CAD build for the part. Positions are in the model's coordinates, mm. A direction names the side the tool comes from. Round coordinates to 2 decimals unless told otherwise and drop trailing zeros. Write each loop counter-clockwise with the first axis right and the second up, starting at its lowest first coordinate (ties: lowest second). Pieces come first, ordered by that corner, then holes. Notation, with made-up numbers: (-7.5, 45) - (45.5, 45) arc R21 ccw to (45.5, 73) - close; hole circle Ø10 at (75, -38). An arc over 180 degrees is marked (long way). Use one line per item in the form item = value. Start each with the question number.
Item 1: Band-saw the part on D-D, the plane x = 18. List the corners of the cut face in (y, z).
Item 2: Tool access for faces 1 (the cylindrical face through (0.73, 3.147, 10.015)), 2 (the flat face through (0, 0, 0)): list every direction of +Z, -Z, +X, -X, +Y, -Y with a clear straight run to the whole face (end or side of a thin tool).
Item 3: Drill centre lines: L1, parallel to Z at x = -5, y = 4.25; L2, parallel to Z at x = -6, y = 5.75; L3, parallel to X at y = 1.25, z = 4.5. Where is each one in solid material? Low to high.
Item 4: Band-saw the part on A-A, the plane y = 2.25. Give the number of separate pieces and of enclosed holes in the cut face, and give its area (3 significant figures).
Item 5: Pin check, flat tips, straight feed: pin 1 (1 mm diameter, centred on y = 0.5, z = 11, fed in from +X); pin 2 (2 mm diameter, centred on x = -5, z = 17, fed in from +Y); pin 3 (1 mm diameter, centred on x = 8, y = 3.5, fed in from -Z); pin 4 (1 mm diameter, centred on x = -19, z = 16, fed in from -Y). Stop position of each tip, or through.
from build123d import *

# Parameters (mm, degrees)
SKETCH1_R           = 50.8
BOSS_EXTRUDE1_DEPTH = 25.4
SKETCH2_R           = 69.85
SKETCH2_R_2         = 50.8
BOSS_EXTRUDE2_DEPTH = 12.7
SKETCH3_R           = 49.53
SKETCH3_R_2         = 47.625
CUT_EXTRUDE1_DEPTH  = 1.1176
CUT_EXTRUDE2_REACH  = 27.4
SKETCH4_R           = 3.175
SKETCH5_R           = 11.43
CUT_EXTRUDE3_DEPTH  = 19.05
SKETCH42_OUTSIDE_W  = 181.538
SKETCH42_OUTSIDE_H  = 181.538
SKETCH42_OUTSIDE_R  = 23.8125
CUT_EXTRUDE9_DEPTH  = 30.48
SKETCH43_R          = 20.6375
CUT_EXTRUDE10_DEPTH = 19.05
SKETCH52_R          = 23.8125
CUT_EXTRUDE11_DEPTH = 19.05
SKETCH55_R          = 1.905
CUT_EXTRUDE12_DEPTH = 7.62
CIRPATTERN1_COUNT   = 8
SKETCH58_R          = 0.9525
CUT_EXTRUDE14_DEPTH = 7.62
CIRPATTERN2_COUNT   = 4
SKETCH59_R          = 0.9525
SKETCH59_R_2        = 1.905
INLET_LID_DEPTH     = 0.03175
SKETCH60_R          = 0.9525
SKETCH60_R_2        = 1.905
OUTLET_LID_DEPTH    = 0.0635


with BuildPart() as part:
    # Sketch1 → Boss-Extrude1 (new body)
    with BuildSketch(Plane(origin=(0, 0, 0), x_dir=(1, 0, 0), z_dir=(0, 1, 0))):
        Circle(SKETCH1_R)
    extrude(amount=BOSS_EXTRUDE1_DEPTH)

    # Sketch2 → Boss-Extrude2 (add)
    with BuildSketch(Plane.XZ):
        Circle(SKETCH2_R)
        Circle(SKETCH2_R_2, mode=Mode.SUBTRACT)
    extrude(amount=-BOSS_EXTRUDE2_DEPTH)

    # Sketch3 → Cut-Extrude1 (cut)
    with BuildSketch(Plane.XZ):
        Circle(SKETCH3_R)
        Circle(SKETCH3_R_2, mode=Mode.SUBTRACT)
    extrude(amount=-CUT_EXTRUDE1_DEPTH, mode=Mode.SUBTRACT)

    # Sketch4 → Cut-Extrude2 (cut, up to next)
    with BuildSketch(Plane.XZ, mode=Mode.PRIVATE) as cut_extrude2_sk1:
        with Locations((0, -59.9186)):
            Circle(SKETCH4_R)
    cut_extrude2_tool1 = extrude(cut_extrude2_sk1.sketch, amount=-CUT_EXTRUDE2_REACH, mode=Mode.PRIVATE) & part.part
    add(cut_extrude2_tool1.solids().sort_by_distance((0, 0, -59.9186))[0], mode=Mode.SUBTRACT)
    # Sketch4 → Cut-Extrude2 (cut, up to next)
    with BuildSketch(Plane.XZ, mode=Mode.PRIVATE) as cut_extrude2_sk2:
        with Locations((-42.368848379, -42.368848379)):
            Circle(SKETCH4_R)
    cut_extrude2_tool2 = extrude(cut_extrude2_sk2.sketch, amount=-CUT_EXTRUDE2_REACH, mode=Mode.PRIVATE) & part.part
    add(cut_extrude2_tool2.solids().sort_by_distance((-42.368848, 0, -42.368848))[0], mode=Mode.SUBTRACT)
    # Sketch4 → Cut-Extrude2 (cut, up to next)
    with BuildSketch(Plane.XZ, mode=Mode.PRIVATE) as cut_extrude2_sk3:
        with Locations((-59.9186, 0)):
            Circle(SKETCH4_R)
    cut_extrude2_tool3 = extrude(cut_extrude2_sk3.sketch, amount=-CUT_EXTRUDE2_REACH, mode=Mode.PRIVATE) & part.part
    add(cut_extrude2_tool3.solids().sort_by_distance((-59.9186, 0, 0))[0], mode=Mode.SUBTRACT)
    # Sketch4 → Cut-Extrude2 (cut, up to next)
    with BuildSketch(Plane.XZ, mode=Mode.PRIVATE) as cut_extrude2_sk4:
        with Locations((-42.368848379, 42.368848379)):
            Circle(SKETCH4_R)
    cut_extrude2_tool4 = extrude(cut_extrude2_sk4.sketch, amount=-CUT_EXTRUDE2_REACH, mode=Mode.PRIVATE) & part.part
    add(cut_extrude2_tool4.solids().sort_by_distance((-42.368848, 0, 42.368848))[0], mode=Mode.SUBTRACT)
    # Sketch4 → Cut-Extrude2 (cut, up to next)
    with BuildSketch(Plane.XZ, mode=Mode.PRIVATE) as cut_extrude2_sk5:
        with Locations((0, 59.9186)):
            Circle(SKETCH4_R)
    cut_extrude2_tool5 = extrude(cut_extrude2_sk5.sketch, amount=-CUT_EXTRUDE2_REACH, mode=Mode.PRIVATE) & part.part
    add(cut_extrude2_tool5.solids().sort_by_distance((0, 0, 59.9186))[0], mode=Mode.SUBTRACT)
    # Sketch4 → Cut-Extrude2 (cut, up to next)
    with BuildSketch(Plane.XZ, mode=Mode.PRIVATE) as cut_extrude2_sk6:
        with Locations((42.368848379, 42.368848379)):
            Circle(SKETCH4_R)
    cut_extrude2_tool6 = extrude(cut_extrude2_sk6.sketch, amount=-CUT_EXTRUDE2_REACH, mode=Mode.PRIVATE) & part.part
    add(cut_extrude2_tool6.solids().sort_by_distance((42.368848, 0, 42.368848))[0], mode=Mode.SUBTRACT)
    # Sketch4 → Cut-Extrude2 (cut, up to next)
    with BuildSketch(Plane.XZ, mode=Mode.PRIVATE) as cut_extrude2_sk7:
        with Locations((59.9186, 0)):
            Circle(SKETCH4_R)
    cut_extrude2_tool7 = extrude(cut_extrude2_sk7.sketch, amount=-CUT_EXTRUDE2_REACH, mode=Mode.PRIVATE) & part.part
    add(cut_extrude2_tool7.solids().sort_by_distance((59.9186, 0, 0))[0], mode=Mode.SUBTRACT)
    # Sketch4 → Cut-Extrude2 (cut, up to next)
    with BuildSketch(Plane.XZ, mode=Mode.PRIVATE) as cut_extrude2_sk8:
        with Locations((42.368848379, -42.368848379)):
            Circle(SKETCH4_R)
    cut_extrude2_tool8 = extrude(cut_extrude2_sk8.sketch, amount=-CUT_EXTRUDE2_REACH, mode=Mode.PRIVATE) & part.part
    add(cut_extrude2_tool8.solids().sort_by_distance((42.368848, 0, -42.368848))[0], mode=Mode.SUBTRACT)

    # Sketch5 → Cut-Extrude3 (cut)
    with BuildSketch(Plane(origin=(0, 25.4, 0), x_dir=(1, 0, 0), z_dir=(0, 1, 0))):
        Circle(SKETCH5_R)
    extrude(amount=-CUT_EXTRUDE3_DEPTH, mode=Mode.SUBTRACT)

    # Sketch42 outside → Cut-Extrude9 (cut)
    with BuildSketch(Plane.XZ):
        Rectangle(SKETCH42_OUTSIDE_W, SKETCH42_OUTSIDE_H)
        Circle(SKETCH42_OUTSIDE_R, mode=Mode.SUBTRACT)
    extrude(amount=-CUT_EXTRUDE9_DEPTH, mode=Mode.SUBTRACT)

    # Sketch43 → Cut-Extrude10 (cut)
    with BuildSketch(Plane(origin=(0, 25.4, 0), x_dir=(1, 0, 0), z_dir=(0, 1, 0))):
        Circle(SKETCH43_R)
    extrude(amount=-CUT_EXTRUDE10_DEPTH, mode=Mode.SUBTRACT)

    # Sketch52 → Cut-Extrude11 (cut)
    with BuildSketch(Plane(origin=(0, 25.4, 0), x_dir=(1, 0, 0), z_dir=(0, 1, 0))):
        Circle(SKETCH52_R)
    extrude(amount=-CUT_EXTRUDE11_DEPTH, mode=Mode.SUBTRACT)

    # Sketch55 → Cut-Extrude12 (cut)
    with BuildSketch(Plane.XZ):
        with Locations((8.255, 0)):
            Circle(SKETCH55_R)
    cut_extrude12 = extrude(amount=-CUT_EXTRUDE12_DEPTH, mode=Mode.SUBTRACT)

    # CirPattern1: Cut-Extrude12 ×8 about axis
    cirpattern1_axis = Axis((0, 0, 0), (0, 1, 0))
    for i in range(1, CIRPATTERN1_COUNT):
        add(cut_extrude12.rotate(cirpattern1_axis, i * 360 / CIRPATTERN1_COUNT), mode=Mode.SUBTRACT)

    # Sketch58 → Cut-Extrude14 (cut)
    with BuildSketch(Plane.XZ):
        with Locations((3.175, 0)):
            Circle(SKETCH58_R)
    cut_extrude14 = extrude(amount=-CUT_EXTRUDE14_DEPTH, mode=Mode.SUBTRACT)

    # CirPattern2: Cut-Extrude14 ×4 about axis
    cirpattern2_axis = Axis((0, 0, 0), (0, 1, 0))
    for i in range(1, CIRPATTERN2_COUNT):
        add(cut_extrude14.rotate(cirpattern2_axis, i * 360 / CIRPATTERN2_COUNT), mode=Mode.SUBTRACT)

    # Sketch59 → Inlet Lid (add, symmetric)
    with BuildSketch(Plane(origin=(0, 6.35, 0), x_dir=(1, 0, 0), z_dir=(0, 1, 0))):
        with Locations((0, -3.175)):
            Circle(SKETCH59_R)
        with Locations((-3.175, 0)):
            Circle(SKETCH59_R)
        with Locations((0, 3.175)):
            Circle(SKETCH59_R)
        with Locations((3.175, 0)):
            Circle(SKETCH59_R)
        with Locations((0, 8.255)):
            Circle(SKETCH59_R_2)
        with Locations((-5.837166479, 5.837166479)):
            Circle(SKETCH59_R_2)
        with Locations((-8.255, 0)):
            Circle(SKETCH59_R_2)
        with Locations((-5.837166479, -5.837166479)):
            Circle(SKETCH59_R_2)
        with Locations((0, -8.255)):
            Circle(SKETCH59_R_2)
        with Locations((5.837166479, -5.837166479)):
            Circle(SKETCH59_R_2)
        with Locations((8.255, 0)):
            Circle(SKETCH59_R_2)
        with Locations((5.837166479, 5.837166479)):
            Circle(SKETCH59_R_2)
    extrude(amount=INLET_LID_DEPTH, both=True)

    # Sketch60 → Outlet Lid (add, symmetric)
    with BuildSketch(Plane.XZ):
        with Locations((0, 3.175)):
            Circle(SKETCH60_R)
        with Locations((-3.175, 0)):
            Circle(SKETCH60_R)
        with Locations((0, -3.175)):
            Circle(SKETCH60_R)
        with Locations((3.175, 0)):
            Circle(SKETCH60_R)
        with Locations((5.837166479, 5.837166479)):
            Circle(SKETCH60_R_2)
        with Locations((0, 8.255)):
            Circle(SKETCH60_R_2)
        with Locations((-5.837166479, 5.837166479)):
            Circle(SKETCH60_R_2)
        with Locations((-8.255, 0)):
            Circle(SKETCH60_R_2)
        with Locations((-5.837166479, -5.837166479)):
            Circle(SKETCH60_R_2)
        with Locations((0, -8.255)):
            Circle(SKETCH60_R_2)
        with Locations((5.837166479, -5.837166479)):
            Circle(SKETCH60_R_2)
        with Locations((8.255, 0)):
            Circle(SKETCH60_R_2)
    extrude(amount=OUTLET_LID_DEPTH, both=True)


solid = part.part
Determined:
q1.outline = (0, -15.59) - (6.35, -15.59) - (6.35, 15.59) - (0, 15.59) - close
q2.face_1 = none
q2.face_2 = -Y
q3.L1 = -23.28 to -7.55, -4.13 to 4.13, 7.55 to 23.28
q3.L2 = -23.04 to -7.74, -3.94 to 3.94, 7.74 to 23.04
q3.L3 = -23.38 to -7.19, -4.48 to 4.48, 7.19 to 23.38
q4.separate_pieces = 1
q4.enclosed_holes = 12
q4.area = 1,680 mm²
q5.pin_1 = 21.37
q5.pin_2 = 6.35
q5.pin_3 = -22.6
q5.pin_4 = through
